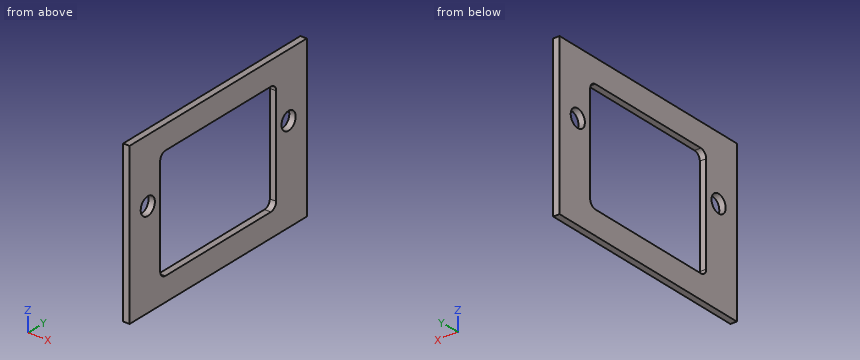
```python
from build123d import *

# Parameters (mm, degrees)
SKETCH1_W           = 25
SKETCH1_H           = 35
BOSS_EXTRUDE1_DEPTH = 1
SKETCH2_R           = 1.4
CUT_EXTRUDE1_DEPTH  = 1


with BuildPart() as part:
    # Sketch1 → Boss-Extrude1 (new body)
    with BuildSketch(Plane(origin=(0, 0, 0), x_dir=(0, 0, -1), z_dir=(1, 0, 0))):
        Rectangle(SKETCH1_W, SKETCH1_H)
    extrude(amount=BOSS_EXTRUDE1_DEPTH)

    # Sketch2 → Cut-Extrude1 (cut)
    with BuildSketch(Plane.ZY):
        with Locations((2.5, 13.9)):
            Circle(SKETCH2_R)
        with Locations((2.5, -13.9)):
            Circle(SKETCH2_R)
        with BuildLine():
            Line((-8.8, 10.4), (-8.8, -10.4))
            ThreePointArc((-8.8, -10.4), (-8.49246212, -11.14246212), (-7.75, -11.45))
            Line((-7.75, -11.45), (7.75, -11.45))
            ThreePointArc((7.75, -11.45), (8.49246212, -11.14246212), (8.8, -10.4))
            Line((8.8, -10.4), (8.8, 10.4))
            ThreePointArc((8.8, 10.4), (8.49246212, 11.14246212), (7.75, 11.45))
            Line((7.75, 11.45), (-7.75, 11.45))
            ThreePointArc((-7.75, 11.45), (-8.49246212, 11.14246212), (-8.8, 10.4))
        make_face()
    extrude(amount=-CUT_EXTRUDE1_DEPTH, mode=Mode.SUBTRACT)


solid = part.part
```
Source: CAD feature listing. Evaluate the final solid. Frame: model axes, mm. Round coordinates to 2 decimals unless told otherwise and drop trailing zeros. Loops run counter-clockwise (first coordinate to the right, second up) from the corner with the lowest first, then second, coordinate; pieces in that order, holes last.
1. Contact query for flat-ended pins moving along their axis: pin 1 (12 mm diameter, centred on y = -11.5, z = -2, fed in from -X); pin 2 (8 mm diameter, centred on y = -1, z = -2, fed in from +X). Output: stop coordinate, or through.
2. Section query D-D on z = 0. Output: boundary loops of the cut face in (x, y), and give its area (3 significant figures).
3. Section query A-A on y = -13.9. Output: boundary loops of the cut face in (x, z).
4. Section query C-C on z = 2.5. Output: boundary loops of the cut face in (x, y), and give its area (3 significant figures).
5. Ray query, L1, parallel to Y at x = 0.6, z = 2.5; L2, parallel to Z at x = 0.95, y = 0; L3, parallel to Y at x = 0.5, z = 1. Return the intervals inside material, ascending.
6. Section query B-B on x = 0.35. Output: boundary loops of the cut face in (y, z).
Answers below:
1. pin 1: stops at x = 0
1. pin 2: passes through
2. outline: (0, -17.5) - (1, -17.5) - (1, -11.45) - (0, -11.45) - close; (0, 11.45) - (1, 11.45) - (1, 17.5) - (0, 17.5) - close
2. area: 12.1 mm2
3. outline: (0, -12.5) - (1, -12.5) - (1, 1.1) - (0, 1.1) - close; (0, 3.9) - (1, 3.9) - (1, 12.5) - (0, 12.5) - close
4. outline: (0, -17.5) - (1, -17.5) - (1, -15.3) - (0, -15.3) - close; (0, -12.5) - (1, -12.5) - (1, -11.45) - (0, -11.45) - close; (0, 11.45) - (1, 11.45) - (1, 12.5) - (0, 12.5) - close; (0, 15.3) - (1, 15.3) - (1, 17.5) - (0, 17.5) - close
4. area: 6.50 mm2
5. L1: y = -17.5 to -15.3, -12.5 to -11.45, 11.45 to 12.5, 15.3 to 17.5
5. L2: z = -12.5 to -8.8, 8.8 to 12.5
5. L3: y = -17.5 to -11.45, 11.45 to 17.5
6. outline: (-17.5, -12.5) - (17.5, -12.5) - (17.5, 12.5) - (-17.5, 12.5) - close; hole circle Ø2.8 at (-13.9, 2.5); hole (-11.45, -7.75) arc R1.05 ccw to (-10.4, -8.8) - (10.4, -8.8) arc R1.05 ccw to (11.45, -7.75) - (11.45, 7.75) arc R1.05 ccw to (10.4, 8.8) - (-10.4, 8.8) arc R1.05 ccw to (-11.45, 7.75) - close; hole circle Ø2.8 at (13.9, 2.5)
